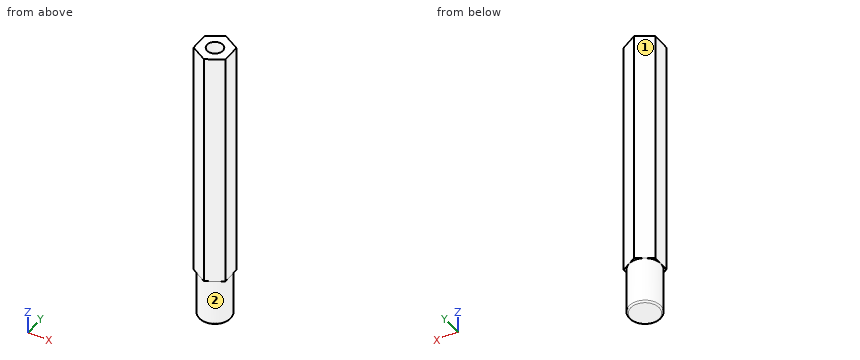
from build123d import *

# Parameters (mm, degrees)
BOSS_EXTRUDE1_DEPTH = 15.333333333
SKETCH2_R           = 0.5
CUT_EXTRUDE1_DEPTH  = 2
SKETCH3_R           = 1
BOSS_EXTRUDE2_DEPTH = 3
FILLET1_R           = 0.1


with BuildPart() as part:
    # Sketch1 → Boss-Extrude1 (new body)
    with BuildSketch(Plane.XY):
        Polygon((0, 1.154700538), (-1, 0.577350269), (-1, -0.577350269), (0, -1.154700538), (1, -0.577350269), (1, 0.577350269), align=None)
    extrude(amount=BOSS_EXTRUDE1_DEPTH)

    # Sketch2 → Cut-Extrude1 (cut)
    with BuildSketch(Plane.XY.offset(15.333333333)):
        Circle(SKETCH2_R)
    extrude(amount=-CUT_EXTRUDE1_DEPTH, mode=Mode.SUBTRACT)

    # Sketch3 → Boss-Extrude2 (add)
    with BuildSketch(Plane(origin=(0, 0, 0), x_dir=(-1, 0, 0), z_dir=(0, 0, -1))):
        Circle(SKETCH3_R)
    extrude(amount=BOSS_EXTRUDE2_DEPTH)

    # Fillet1
    fillet1_edges = [part.edges().sort_by_distance(p)[0] for p in [
        (1, 0, -3),
    ]]
    fillet(fillet1_edges, radius=FILLET1_R)


solid = part.part
Read the model definition and answer for the solid it produces. Units are mm, in the model's axes. Face numbers are marked on the shaded views. A direction names the side the tool comes from. Round coordinates to 2 decimals unless told otherwise and drop trailing zeros. Order: outer loops, then holes, each group sorted by start corner. A loop starts at its lowest first (then second) coordinate and runs counter-clockwise, first axis right, second up.
1) For the marked faces 1 and 2, determine the directions among +Z, -Z, +X, -X, +Y, -Y from which every point of the face is accessible in a straight line to the end or side of a thin tool.
2) The part is cut by section A-A on z = 6.5. Write down the section's boundary in (x, y).
3) Straight lines are drawn through the part: L1, parallel to Z at x = 0.6, y = -0.7; L2, parallel to Y at x = 0.5, z = 5.5; L3, parallel to Y at x = 0.35, z = 11.25. For each, find the intervals that lie inside material, in ascending order.
Resolved:
1. face 1: +Z, -Z, -X, +Y
1. face 2: -Z
2. outline: (-1, -0.58) - (0, -1.15) - (1, -0.58) - (1, 0.58) - (0, 1.15) - (-1, 0.58) - close
3. L1: z = -3 to 15.33
3. L2: y = -0.87 to 0.87
3. L3: y = -0.95 to 0.95
